from build123d import *

# Parameters (mm, degrees)
SKETCH1_R           = 76.2
SKETCH1_R_2         = 3.175
SKETCH1_R_3         = 6.35
BOSS_EXTRUDE1_DEPTH = 2.54


with BuildPart() as part:
    # Sketch1 → Boss-Extrude1 (new body)
    with BuildSketch(Plane(origin=(0, 0, 0), x_dir=(1, 0, 0), z_dir=(0, 1, 0))):
        with Locations(Location((0, 0, 0), (0, 0, 270))):
            Circle(SKETCH1_R)
        with Locations(Location((-16.51, 57.404, 0), (0, 0, 270))):
            Circle(SKETCH1_R_2, mode=Mode.SUBTRACT)
        with Locations(Location((16.51, 57.404, 0), (0, 0, 270))):
            Circle(SKETCH1_R_2, mode=Mode.SUBTRACT)
        with Locations(Location((57.404, -16.51, 0), (0, 0, 270))):
            Circle(SKETCH1_R_2, mode=Mode.SUBTRACT)
        with Locations(Location((57.404, 16.51, 0), (0, 0, 270))):
            Circle(SKETCH1_R_2, mode=Mode.SUBTRACT)
        with Locations(Location((-16.51, -57.404, 0), (0, 0, 270))):
            Circle(SKETCH1_R_2, mode=Mode.SUBTRACT)
        with Locations(Location((16.51, -57.404, 0), (0, 0, 270))):
            Circle(SKETCH1_R_2, mode=Mode.SUBTRACT)
        with Locations(Location((-57.404, 16.51, 0), (0, 0, 270))):
            Circle(SKETCH1_R_2, mode=Mode.SUBTRACT)
        with Locations(Location((-57.404, -16.51, 0), (0, 0, 270))):
            Circle(SKETCH1_R_2, mode=Mode.SUBTRACT)
        with Locations(Location((0, 0, 0), (0, 0, 270))):
            Circle(SKETCH1_R_3, mode=Mode.SUBTRACT)
        with BuildLine():
            Line((-3.099389971, 12.315996988), (-3.099389971, 50.705362456))
            ThreePointArc((-3.099389971, 50.705362456), (-35.921024484, 35.921024484), (-50.705362456, 3.099389971))
            Line((-50.705362456, 3.099389971), (-12.315996988, 3.099389971))
            ThreePointArc((-12.315996988, 3.099389971), (-8.980256121, 8.980256121), (-3.099389971, 12.315996988))
        make_face(mode=Mode.SUBTRACT)
        with BuildLine():
            Line((3.099389971, 12.315996988), (3.099389971, 50.705362456))
            ThreePointArc((3.099389971, 50.705362456), (35.921024484, 35.921024484), (50.705362456, 3.099389971))
            Line((50.705362456, 3.099389971), (12.315996988, 3.099389971))
            ThreePointArc((12.315996988, 3.099389971), (8.980256121, 8.980256121), (3.099389971, 12.315996988))
        make_face(mode=Mode.SUBTRACT)
        with BuildLine():
            Line((12.315996988, -3.099389971), (50.705362456, -3.099389971))
            ThreePointArc((50.705362456, -3.099389971), (35.921024484, -35.921024484), (3.099389971, -50.705362456))
            Line((3.099389971, -50.705362456), (3.099389971, -12.315996988))
            ThreePointArc((3.099389971, -12.315996988), (8.980256121, -8.980256121), (12.315996988, -3.099389971))
        make_face(mode=Mode.SUBTRACT)
        with BuildLine():
            Line((-3.099389971, -12.315996988), (-3.099389971, -50.705362456))
            ThreePointArc((-3.099389971, -50.705362456), (-35.921024484, -35.921024484), (-50.705362456, -3.099389971))
            Line((-50.705362456, -3.099389971), (-12.315996988, -3.099389971))
            ThreePointArc((-12.315996988, -3.099389971), (-8.980256121, -8.980256121), (-3.099389971, -12.315996988))
        make_face(mode=Mode.SUBTRACT)
    extrude(amount=BOSS_EXTRUDE1_DEPTH)


solid = part.part
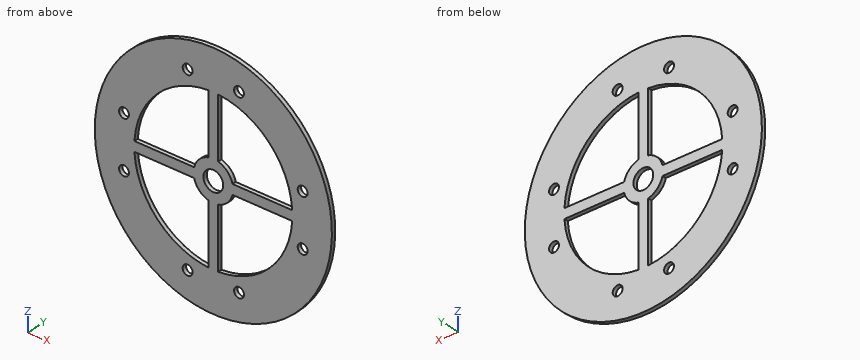
Read the model definition and answer for the solid it produces. Units are mm, in the model's axes. Give positions to 0.01 mm unless a question says otherwise; leave off trailing zeros. Loops run counter-clockwise (first coordinate to the right, second up) from the corner with the lowest first, then second, coordinate; pieces in that order, holes last. Notation, with made-up numbers: M 43,56 L 98,56 A6 ccw 98,67 Z; hole C 2,71 d2. An arc over 180 degrees is marked long. Write each question's results on one line, items separated by ' | '.
1. Section C-C on z = -22 is taken. Give the vertices of the cut face in (x, y), plus the area to 3 significant figures.
Values:
outline: M -72.96,0 L -45.79,0 L -45.79,2.54 L -72.96,2.54 Z; M -3.1,0 L 3.1,0 L 3.1,2.54 L -3.1,2.54 Z; M 45.79,0 L 72.96,0 L 72.96,2.54 L 45.79,2.54 Z | area: 154 mm^2
2. Straight lines are drawn through the part: line 1 (X direction, y = 2.35, z = 0); line 2 (Z direction, x = -21, y = 0.7); line 3 (Z direction, x = -16, y = 2.15). For each, find the intervals that lie inside material, in ascending order. Write a range as [from, to].
Values:
line 1: x = [-76.2, -6.35], [6.35, 76.2] | line 2: z = [-73.25, -46.26], [-3.1, 3.1], [46.26, 73.25] | line 3: z = [-74.5, -60.54], [-54.27, -48.21], [-3.1, 3.1], [48.21, 54.27], [60.54, 74.5]
3. Section D-D on y = 1.15 is taken. State how many separate pieces and enclosed holes the cut face has, plus the area to 3 significant figures.
Values:
separate pieces: 1 | enclosed holes: 13 | area: 11,200 mm^2
4. Section A-A on z = 0 is taken. Give the vertices of the cut face in (x, y).
Values:
outline: M -76.2,0 L -6.35,0 L -6.35,2.54 L -76.2,2.54 Z; M 6.35,0 L 76.2,0 L 76.2,2.54 L 6.35,2.54 Z
5. Section B-B on x = -43.5 is taken. Give the vertices of the cut face in (y, z), plus the area to 3 significant figures.
Values:
outline: M 0,-62.56 L 2.54,-62.56 L 2.54,-26.24 L 0,-26.24 Z; M 0,-3.1 L 2.54,-3.1 L 2.54,3.1 L 0,3.1 Z; M 0,26.24 L 2.54,26.24 L 2.54,62.56 L 0,62.56 Z | area: 200 mm^2
6. Given pin 1 (0.8 mm diameter, centred on x = 32.5, y = 2, fed in from -Z); pin 2 (0.8 mm diameter, centred on x = -26, y = 1.5, fed in from +Z); pin 3 (0.8 mm diameter, centred on y = 2, z = 23, fed in from -X), each flat-ended and moving along its own axis, determine where each tip first touches the part or whether it passes through.
Values:
pin 1: stops at z = -69.11 | pin 2: stops at z = 71.77 | pin 3: stops at x = -72.77
